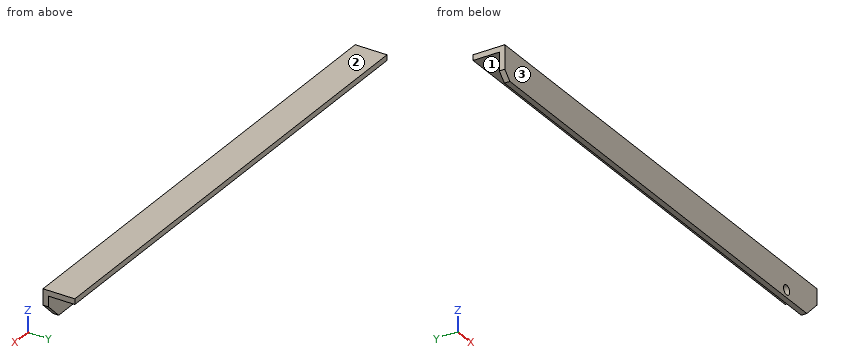
```python
from build123d import *

# Parameters (mm, degrees)
BOSS_EXTRUDE1_DEPTH = 308
SKETCH2_R           = 3
CUT_EXTRUDE1_DEPTH  = 310.295974756


with BuildPart() as part:
    # Sketch1 → Boss-Extrude1 (new body)
    with BuildSketch(Plane(origin=(0, 0, 0), x_dir=(0, 0, -1), z_dir=(1, 0, 0))):
        Polygon((0, 0), (20, 0), (20, 3.461178467), (3.461178467, 3.461178467), (3.461178467, 20), (0, 20), align=None)
    extrude(amount=BOSS_EXTRUDE1_DEPTH)

    # Sketch2 → Cut-Extrude1 (cut, through all)
    with BuildSketch(Plane(origin=(0, 0, 0), x_dir=(1, 0, 0), z_dir=(0, 1, 0))):
        with Locations(Location((278, 15.25, 0), (0, 0, 90))):
            Circle(SKETCH2_R)
        Polygon((308, 10), (298, 20), (308, 20), align=None)
        Polygon((0, 20), (5, 20), (0, 15), align=None)
    extrude(amount=CUT_EXTRUDE1_DEPTH, mode=Mode.SUBTRACT)


solid = part.part
```
CAD build for the part. Positions are in the model's coordinates, mm. Face numbers are marked on the shaded views. Coordinates: 2 decimals unless noted, no trailing zeros. Write each loop counter-clockwise with the first axis right and the second up, starting at its lowest first coordinate (ties: lowest second). Pieces come first, ordered by that corner, then holes.
(1) Two-plate mould, pull along Z, no slides. Class the marked faces 1, 2 and 3: +Z half, -Z half, draft (parallel to the pull), parting line (faces both ways), or undercut.
(2) Cut at A-A, the plane x = 278. List the corners of the cut face in (y, z), and give its area (3 significant figures).
(3) Flat gauge pins, fed straight in: pin 1 (8 mm diameter, centred on x = 231.5, z = -7.5, fed in from +Y); pin 2 (5.5 mm diameter, centred on x = 278, z = -15.25, fed in from +Y); pin 3 (5 mm diameter, centred on x = 211.5, y = 8, fed in from -Z). Where does each tip first touch, or does it go through?
(4) Cut at C-C, the plane y = 13.75. List the corners of the cut face in (x, z).
(5) Drill centre lines: probe 1 along Z at (x, y) = (278, 1.3); probe 2 along Y at (x, z) = (68, -14.5); probe 3 along X at (y, z) = (1.4, -15.25). Where is each one in solid material? Low to high.
(6) Cut at B-B, the plane x = 199. List the corners of the cut face in (y, z).
Geometry says:
1. face 1: -Z half
1. face 2: +Z half
1. face 3: draft
2. outline: (0, -20) - (3.46, -20) - (3.46, -18.25) - (0, -18.25) - close; (0, -12.25) - (3.46, -12.25) - (3.46, -3.46) - (20, -3.46) - (20, 0) - (0, 0) - close
2. area: 106 mm2
3. pin 1: stops at y = 3.46
3. pin 2: passes through
3. pin 3: stops at z = -3.46
4. outline: (0, -3.46) - (308, -3.46) - (308, 0) - (0, 0) - close
5. probe 1: z = -20 to -18.25, -12.25 to 0
5. probe 2: y = 0 to 3.46
5. probe 3: x = 0.25 to 275, 281 to 302.75
6. outline: (0, -20) - (3.46, -20) - (3.46, -3.46) - (20, -3.46) - (20, 0) - (0, 0) - close
